CAD build for the part. Positions are in the model's coordinates, mm. Round coordinates to 2 decimals unless told otherwise and drop trailing zeros.
```python
from build123d import *

# Parameters (mm, degrees)
F0_R     = 3.175
F1_DEPTH = 6.35


with BuildPart() as f1:
    # F0 (on Front) → F1 (new body)
    with BuildSketch(Plane.XZ):
        with BuildLine():
            add(Edge.make_bspline(
                [(-6.0602840723, 31.8534711944), (-8.9123209928, 26.7616721507), (-9.5678060072, 21.1194401062), (-10.7354209084, 5.442497338), (-7.3669134372, -2.9550791291)],
                knots=[0, 0, 0, 0, 0.4184743156, 1, 1, 1, 1], degree=3))
            ThreePointArc((-7.3669134372, -2.9550791291), (-1.63587801, -7.7670978741), (5.5491886165, -5.6754217419))
            add(Edge.make_bspline(
                [(24.4385115585, 17.1715788698), (22.5209788834, 13.5742014085), (17.275688011, 6.7190147021), (11.0943717174, -0.2535749894), (5.5491886165, -5.6754217419)],
                knots=[0.1380846356, 0.1380846356, 0.1380846356, 0.1380846356, 0.4828720967, 1, 1, 1, 1], degree=3))
            ThreePointArc((24.4385115585, 17.1715788698), (24.7420563147, 19.326379645), (23.5868786889, 21.1705245559))
            add(Edge.make_bspline(
                [(-3.074806905, 33.4695786248), (3.1958280854, 33.0431476028), (12.0935678521, 29.2874679133), (18.4108124786, 25.1994105978), (23.5868786889, 21.1705245559)],
                knots=[0, 0, 0, 0, 0.5068320595, 1, 1, 1, 1], degree=3))
            ThreePointArc((-3.074806905, 33.4695786248), (-4.8016804973, 33.0940485831), (-6.0602840723, 31.8534711944))
        make_face()
        Circle(F0_R, mode=Mode.SUBTRACT)
    extrude(amount=F1_DEPTH)


solid = f1.part
```
1. Pin check, flat tips, straight feed: P1, Ø5.5, axis at x = 0, z = 0, coming from the -Y side; P2, Ø1.5, axis at y = -3, z = 5.5, coming from the -X side; P3, Ø1, axis at x = 10.5, y = -4, coming from the -Z side; P4, Ø2, axis at y = -4.5, z = 27.5, coming from the +X side. Stop position of each tip, or through.
2. Mould opens along Z. For faces 1 (the face through (24.748, -3.131, 19.296)), 2 (the face through (3, -6.35, 13)), 3 (the face through (-0.69, -3.13, -3.1)) say: released by +Z, released by -Z, zero draft, split by the parting line, or undercut.
3. Drill centre lines: line 1 (Z direction, x = 0, y = -2.25) (1 decimal); line 2 (Z direction, x = 2, y = -5.25); line 3 (X direction, y = -0.5, z = 14). Where is each one in solid material? Low to high.
Outcome:
1. P1: passes through
1. P2: stops at x = -9.63
1. P3: stops at z = -1.19
1. P4: stops at x = 16.18
2. face 1: split by the parting line
2. face 2: zero draft
2. face 3: undercut
3. line 1: z = -7.9 to -3.2, 3.2 to 33.1
3. line 2: z = -7.68 to -2.47, 2.47 to 32.75
3. line 3: x = -9.95 to 22.57
